Study the drawing (mm; zero at the part's minimum x, y, z) and answer. Coordinates: 2 decimals unless noted, no trailing zeros. Order: outer loops, then holes, each group sorted by start corner. A loop starts at its lowest first (then second) coordinate and runs counter-clockwise, first axis right, second up.
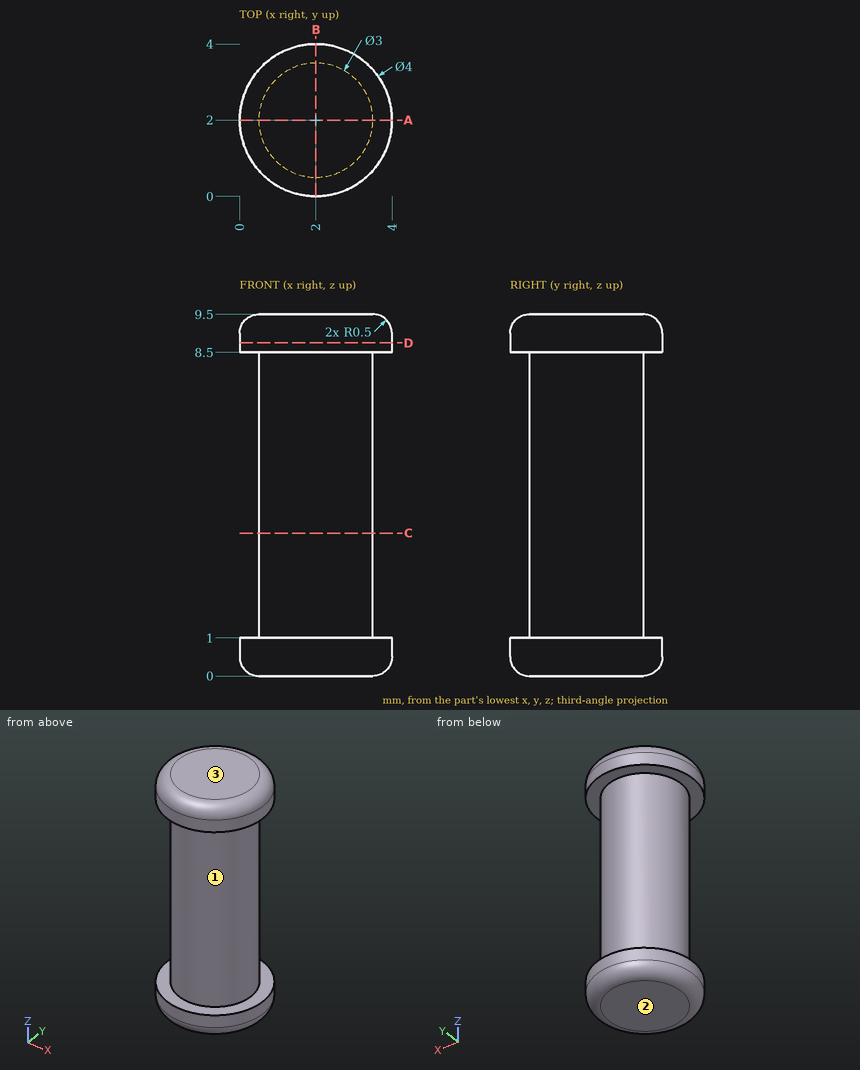
(1) Consider line 1 (Z direction, x = 0.5, y = 1.5); line 2 (Z direction, x = 2.6, y = 0.2); line 3 (Y direction, x = 1.95, z = 5). Determine where each line is inside the solid, lowest interval first.
(2) Find section C-C (z = 3.75). Write down the section's boundary in (x, y), and give its area (3 significant figures).
(3) Find section A-A (y = 2). Write down the section's boundary in (x, z).
(4) Find section D-D (z = 8.75). Write down the section's boundary in (x, y).
(5) The mould has two halves that part along Z. Classify the marked faces 1, 2 and 3: released by +Z, released by -Z, zero draft, split by the parting line, or undercut.
Findings below:
1. line 1: z = 0.01 to 1, 8.5 to 9.49
1. line 2: z = 0.2 to 1, 8.5 to 9.3
1. line 3: y = 0.5 to 3.5
2. outline: circle Ø3 at (2, 2)
2. area: 7.07 mm2
3. outline: (0, 0.5) arc R0.5 ccw to (0.5, 0) - (3.5, 0) arc R0.5 ccw to (4, 0.5) - (4, 1) - (3.5, 1) - (3.5, 8.5) - (4, 8.5) - (4, 9) arc R0.5 ccw to (3.5, 9.5) - (0.5, 9.5) arc R0.5 ccw to (0, 9) - (0, 8.5) - (0.5, 8.5) - (0.5, 1) - (0, 1) - close
4. outline: circle Ø4 at (2, 2)
5. face 1: undercut
5. face 2: released by -Z
5. face 3: released by +Z
